Can you work these out from the model? Positions are in its coordinate system, mm. Coordinates: 2 decimals unless noted, no trailing zeros. Write each loop counter-clockwise with the first axis right and the second up, starting at its lowest first coordinate (ties: lowest second). Pieces come first, ordered by that corner, then holes.
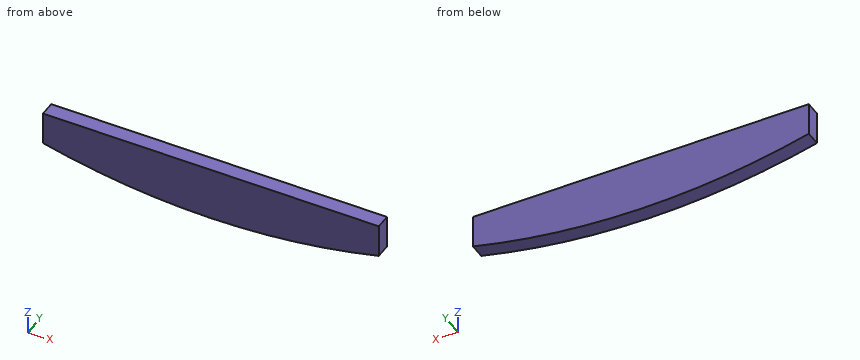
```python
from build123d import *

# Parameters (mm, degrees)
CYLINDER002_R          = 630
CYLINDER002_DEPTH      = 15
CYLINDER002_ROLL_ANGLE = 90
BOX025_W               = 50
BOX025_H               = 15
BOX025_DEPTH           = 310
BOX025_PITCH_ANGLE     = 90


with BuildPart() as obj1:
    # Cylinder002 → Cylinder002 (new body)
    with BuildSketch(Plane.XY):
        Circle(CYLINDER002_R)
    extrude(amount=CYLINDER002_DEPTH)


with BuildPart() as obj1_1:
    # Cylinder002 roll: moved
    add(obj1.part.rotate(Axis((0, 0, 0), (1, 0, 0)), CYLINDER002_ROLL_ANGLE))


with BuildPart() as obj1_2:
    # Cylinder002 placement: moved
    add(obj1_1.part.moved(Location((400, 118, 710))))


with BuildPart() as obj2:
    # Box025 → Box025 (new body)
    with BuildSketch(Plane.XY):
        with Locations((25, 7.5)):
            Rectangle(BOX025_W, BOX025_H)
    extrude(amount=BOX025_DEPTH)


with BuildPart() as obj2_1:
    # Box025 pitch: moved
    add(obj2.part.rotate(Axis((0, 0, 0), (0, 1, 0)), BOX025_PITCH_ANGLE))


with BuildPart() as obj2_2:
    # Box025 placement: moved
    add(obj2_1.part.moved(Location((245, 102, 130))))

    # Common: intersect obj1
    add(obj1_2.part, mode=Mode.INTERSECT)


solid = obj2_2.part
```
1. If we section it at B-B, the plane x = 514: List the corners of the cut face in (y, z) for me, plus the area to 3 significant figures.
2. If we section it at A-A, the plane y = 112.75: List the corners of the cut face in (x, z) for me.
3. If I drill on L1, parallel to Z at x = 394.5, y = 107.75; L2, parallel to Z at x = 337.5, y = 104.75, over which ranges is the centre line in solid material (lowest first)?
Answers:
1. outline: (103, 90.4) - (117, 90.4) - (117, 130) - (103, 130) - close
1. area: 554 mm2
2. outline: (245, 99.37) arc R630 ccw to (555, 99.37) - (555, 130) - (245, 130) - close
3. L1: z = 80.02 to 130
3. L2: z = 83.11 to 130
